```python
from build123d import *

# Parameters (mm, degrees)
F1_DEPTH = 16
F2_SIZE  = 15.99999


# Not quite as in the source:
# - a fillet or chamfer is up to 0.001 mm smaller than in the source, because OpenCascade refuses the exact size


with BuildPart() as f1:
    # F0 (on Right) → F1 (new body)
    with BuildSketch(Plane.YZ):
        Polygon((0, 59.6152422707), (0, 0), (300, 0), (300, 140), align=None)
    extrude(amount=F1_DEPTH)

    # F2 (size 16 in the source; OpenCascade refuses exactly that, so slightly less here)
    f2_edges = [f1.edges().sort_by_distance(p)[0] for p in [
        (0, 0, 29.807621),
        (0, 150, 0),
    ]]
    chamfer(f2_edges, length=F2_SIZE)


solid = f1.part
```
Model file for the job. Use its own axes, mm. Coordinates: 2 decimals unless noted, no trailing zeros. Write each loop counter-clockwise with the first axis right and the second up, starting at its lowest first coordinate (ties: lowest second). Pieces come first, ordered by that corner, then holes. Notation, with made-up numbers: (46.5, 0) - (88.5, 0) arc R30 ccw to (88.5, 36) - close; hole circle Ø11 at (-14, -18.75). An arc over 180 degrees is marked (long way). One line per question, with ' | ' between items. Start each with the question number.
Q1. Drill centre lines: line 1 (Z direction, x = 10, y = 63); line 2 (Z direction, x = 1.5, y = 149); line 3 (Y direction, x = 5, z = 30). Where is each one in solid material? Low to high. Write a range as [from, to].
Q2. Cut at D-D, the plane z = 100. List the corners of the cut face in (x, y).
Q3. Cut at C-C, the plane x = 3.5. List the corners of the cut face in (y, z).
Q4. Pin check, flat tip, straight feed: pin 1 (6 mm diameter, centred on x = 11.5, y = 206, fed in from -Z). Stop position of the tip, or through.
Answer below:
1) line 1: [6, 76.5] | line 2: [14.5, 99.54] | line 3: [11, 300]
2) outline: (0, 150.72) - (16, 150.72) - (16, 300) - (0, 300) - close
3) outline: (12.5, 12.5) - (300, 12.5) - (300, 140) - (12.5, 62.96) - close
4) pin 1: z = 1.5
